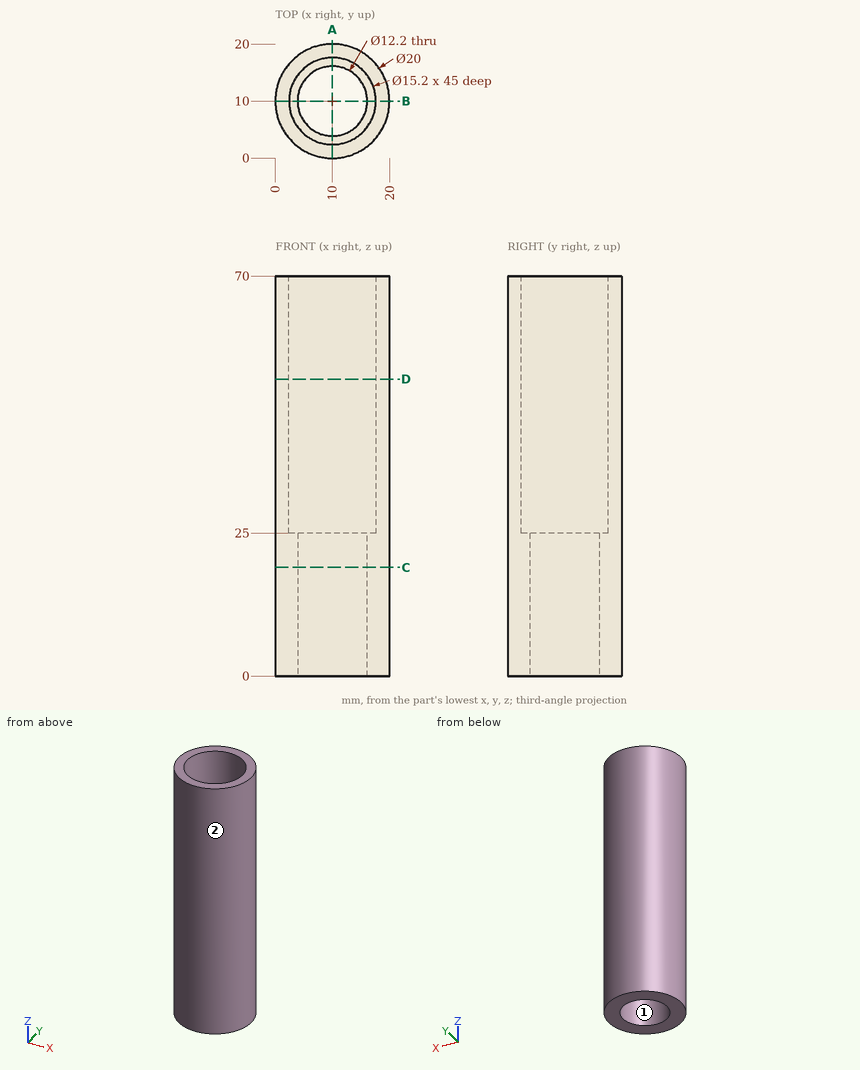
Answer from the drawing. Dimensions are ordinates in mm from the lowest x, y and z of the part. Coordinates: 2 decimals unless noted, no trailing zeros. Write each loop counter-clockwise with the first axis right and the second up, starting at its lowest first coordinate (ties: lowest second). Pieces come first, ordered by that corner, then holes. Notation, with made-up numbers: (55.5, 7.5) - (85.5, 7.5) arc R26 cw to (85.5, 23.5) - close; hole circle Ø10 at (-17, -25). An arc over 180 degrees is marked (long way). Return JSON: item names as keys, results as strings. Group by question number.
Q1. The part is cut by section A-A on x = 10. Write down the section's boundary in (y, z), and give its area (3 significant figures).
Q2. The part is cut by section C-C on z = 19. Write down the section's boundary in (x, y), and give its area (3 significant figures).
Q3. Find the intervals of material crossed by line 1 along Y through (x, z) = (10, 35); line 2 along Y through (x, z) = (10, 5.75); line 3 along X through (y, z) = (14.5, 38.5), in increasing order. Write a range as [from, to].
Q4. The part is cut by section D-D on z = 52. Write down the section's boundary in (x, y).
Q5. Flat-ended cylindrical pins translate along their axes: pin 1 Ø2 at (x, y) = (7, 4.5) entering from +Z; pin 2 Ø6 at (y, z) = (3.5, 54) entering from -X; pin 3 Ø2 at (y, z) = (5, 22.5) entering from +X. Find the tip coordinate at first contact, or state that the pin passes through.
Q6. For a pull along X with two mould halves and no side action, classify the marked faces 1 and 2 as +X half, -X half, draft (parallel to the pull), parting line (faces both ways), or undercut.
Evaluation:
{
 "1": {"outline": "(0, 0) - (3.9, 0) - (3.9, 25) - (2.4, 25) - (2.4, 70) - (0, 70) - close; (16.1, 0) - (20, 0) - (20, 70) - (17.6, 70) - (17.6, 25) - (16.1, 25) - close", "area": "411 mm2"},
 "2": {"outline": "circle Ø20 at (10, 10); hole circle Ø12.2 at (10, 10)", "area": "197 mm2"},
 "3": {"line 1": "y = [0, 2.4], [17.6, 20]", "line 2": "y = [0, 3.9], [16.1, 20]", "line 3": "x = [1.07, 3.88], [16.12, 18.93]"},
 "4": {"outline": "circle Ø20 at (10, 10); hole circle Ø15.2 at (10, 10)"},
 "5": {"pin 1": "stops at z = 25", "pin 2": "stops at x = 0.63", "pin 3": "stops at x = 19.17"},
 "6": {"face 1": "undercut", "face 2": "parting line"}
}
